Here's how the part is built. I have some questions about the finished solid (model axes, mm). Round coordinates to 2 decimals unless told otherwise and drop trailing zeros. Order: outer loops, then holes, each group sorted by start corner. A loop starts at its lowest first (then second) coordinate and runs counter-clockwise, first axis right, second up.
```python
from build123d import *

# Parameters (mm, degrees)
SKETCH_3_R          = 35
EXTRUDE_1_DEPTH     = 3.5
CUT_EXTRUDE_5_DEPTH = 1.2
SKETCH_4_W          = 5
SKETCH_4_H          = 0.8
CUT_EXTRUDE_6_DEPTH = 50.621064076
SKETCH_5_R          = 2.4
CUT_EXTRUDE_7_DEPTH = 50.619451831


with BuildPart() as part:
    # Sketch 3 → Extrude 1 (new body)
    with BuildSketch(Plane(origin=(0, 0, 0), x_dir=(1, 0, 0), z_dir=(0, 1, 0))):
        with Locations(Location((0, 0, 0), (0, 0, 270))):
            Circle(SKETCH_3_R)
    extrude(amount=EXTRUDE_1_DEPTH)

    # Sketch 1 → Cut-Extrude 5 (cut)
    with BuildSketch(Plane(origin=(0, 0, 0), x_dir=(1, 0, 0), z_dir=(0, 1, 0))):
        Polygon((12.628553268, -30.488024573), (30.488024573, -12.628553268), (30.488024573, 12.628553268), (12.628553268, 30.488024573), (-12.628553268, 30.488024573), (-30.488024573, 12.628553268), (-30.488024573, -12.628553268), (-12.628553268, -30.488024573), align=None)
        Polygon((12.214339706, -29.488024573), (29.488024573, -12.214339706), (29.488024573, 12.214339706), (12.214339706, 29.488024573), (-12.214339706, 29.488024573), (-29.488024573, 12.214339706), (-29.488024573, -12.214339706), (-12.214339706, -29.488024573), align=None, mode=Mode.SUBTRACT)
        Polygon((-10.715136106, -25.86862691), (10.715136106, -25.86862691), (25.86862691, -10.715136106), (25.86862691, 10.715136106), (10.715136106, 25.86862691), (-10.715136106, 25.86862691), (-25.86862691, 10.715136106), (-25.86862691, -10.715136106), align=None)
        Polygon((-10.300922544, -24.86862691), (10.300922544, -24.86862691), (24.86862691, -10.300922544), (24.86862691, 10.300922544), (10.300922544, 24.86862691), (-10.300922544, 24.86862691), (-24.86862691, 10.300922544), (-24.86862691, -10.300922544), align=None, mode=Mode.SUBTRACT)
        Polygon((8.706048086, -21.018259365), (21.018259365, -8.706048086), (21.018259365, 8.706048086), (8.706048086, 21.018259365), (-8.706048086, 21.018259365), (-21.018259365, 8.706048086), (-21.018259365, -8.706048086), (-8.706048086, -21.018259365), align=None)
        Polygon((8.291834524, -20.018259365), (20.018259365, -8.291834524), (20.018259365, 8.291834524), (8.291834524, 20.018259365), (-8.291834524, 20.018259365), (-20.018259365, 8.291834524), (-20.018259365, -8.291834524), (-8.291834524, -20.018259365), align=None, mode=Mode.SUBTRACT)
        Polygon((6.888301783, -16.629831585), (16.629831585, -6.888301783), (16.629831585, 6.888301783), (6.888301783, 16.629831585), (-6.888301783, 16.629831585), (-16.629831585, 6.888301783), (-16.629831585, -6.888301783), (-6.888301783, -16.629831585), align=None)
        Polygon((6.47408822, -15.629831585), (15.629831585, -6.47408822), (15.629831585, 6.47408822), (6.47408822, 15.629831585), (-6.47408822, 15.629831585), (-15.629831585, 6.47408822), (-15.629831585, -6.47408822), (-6.47408822, -15.629831585), align=None, mode=Mode.SUBTRACT)
    extrude(amount=CUT_EXTRUDE_5_DEPTH, mode=Mode.SUBTRACT)

    # Sketch 4 → Cut-Extrude 6 (cut, through all)
    with BuildSketch(Plane(origin=(0, 3.5, 0), x_dir=(1, 0, 0), z_dir=(0, 1, 0))):
        with Locations((-34.5, 0)):
            Rectangle(SKETCH_4_W, SKETCH_4_H)
        with Locations((34.5, 0)):
            Rectangle(SKETCH_4_W, SKETCH_4_H)
    extrude(amount=-CUT_EXTRUDE_6_DEPTH, mode=Mode.SUBTRACT)

    # Sketch 5 → Cut-Extrude 7 (cut, through all)
    with BuildSketch(Plane(origin=(0, 3.5, 0), x_dir=(1, 0, 0), z_dir=(0, 1, 0))):
        with Locations(Location((0, 0, 0), (0, 0, 270))):
            Circle(SKETCH_5_R)
    extrude(amount=-CUT_EXTRUDE_7_DEPTH, mode=Mode.SUBTRACT)


solid = part.part
```
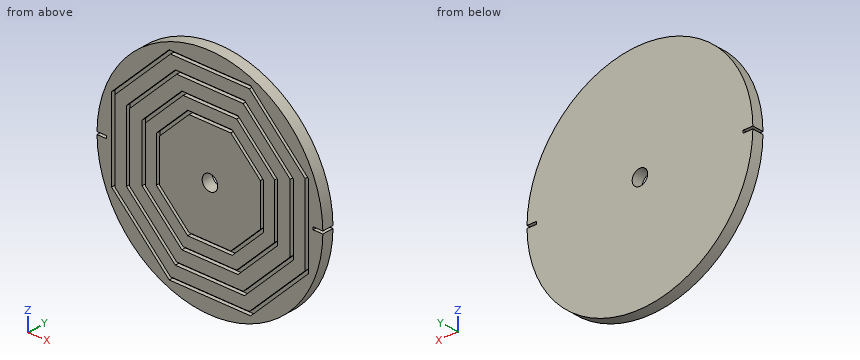
1) I'm going to push flat-ended pins straight in: pin 1 (1 mm diameter, centred on x = 3.5, y = 0.5, fed in from +Z); pin 2 (2 mm diameter, centred on x = -28, y = 2, fed in from -Z); pin 3 (1 mm diameter, centred on x = -23, y = 2.5, fed in from +Z). Where does each tip first touch, or does it pass through?
2) If we section it at B-B (z = -23.5): Write out the boundary of the cut face in (x, y).
3) I need wall thicknesses on line 1 (X direction, y = 1.7, z = 0); line 2 (X direction, y = 0.95, z = 23); line 3 (Z direction, x = 32.5, y = 0.65). Which ranges of each line are inside material? Lowest first, please.
4) If we section it at C-C (z = 19): Write out the boundary of the cut face in (x, y).
Solutions:
1. pin 1: stops at z = 34.87
1. pin 2: stops at z = -22.27
1. pin 3: stops at z = 26.81
2. outline: (-25.94, 0) - (-19.62, 0) - (-19.62, 1.2) - (-18.2, 1.2) - (-18.2, 0) - (-13.08, 0) - (-13.08, 1.2) - (-11.67, 1.2) - (-11.67, 0) - (11.67, 0) - (11.67, 1.2) - (13.08, 1.2) - (13.08, 0) - (18.2, 0) - (18.2, 1.2) - (19.62, 1.2) - (19.62, 0) - (25.94, 0) - (25.94, 3.5) - (-25.94, 3.5) - close
3. line 1: x = -32 to -2.4, 2.4 to 32
3. line 2: x = -26.38 to -20.12, -18.7 to -13.58, -12.17 to 12.17, 13.58 to 18.7, 20.12 to 26.38
3. line 3: z = -12.99 to -0.4, 0.4 to 12.99
4. outline: (-29.39, 0) - (-24.12, 0) - (-24.12, 1.2) - (-22.7, 1.2) - (-22.7, 0) - (-17.58, 0) - (-17.58, 1.2) - (-16.17, 1.2) - (-16.17, 0) - (-10.72, 0) - (-10.72, 1.2) - (-9.31, 1.2) - (-9.31, 0) - (9.31, 0) - (9.31, 1.2) - (10.72, 1.2) - (10.72, 0) - (16.17, 0) - (16.17, 1.2) - (17.58, 1.2) - (17.58, 0) - (22.7, 0) - (22.7, 1.2) - (24.12, 1.2) - (24.12, 0) - (29.39, 0) - (29.39, 3.5) - (-29.39, 3.5) - close
